from build123d import *

# Parameters (mm, degrees)
BOSS_EXTRU_1_DEPTH           = 35
ESQUISSE2_W                  = 30
ESQUISSE2_H                  = 5.1
ENL_V_MAT_EXTRU_1_DEPTH      = 10
ENL_V_MAT_EXTRU_2_DEPTH      = 38.178656511
ENL_V_MAT_EXTRU_2_DEPTH_BACK = 38.178656511
ESQUISSE3_R                  = 2.05
CONG_1_R                     = 1.5


with BuildPart() as part:
    # Esquisse1 → Boss.-Extru.1 (new body)
    with BuildSketch(Plane(origin=(0, 0, 0), x_dir=(0, 0, -1), z_dir=(1, 0, 0))):
        with BuildLine():
            Line((6, 7.5), (-6, 7.5))
            ThreePointArc((-6, 7.5), (-7.060660172, 7.060660172), (-7.5, 6))
            Line((-7.5, 6), (-7.5, -6))
            ThreePointArc((-7.5, -6), (-7.060660172, -7.060660172), (-6, -7.5))
            Line((-6, -7.5), (6, -7.5))
            ThreePointArc((6, -7.5), (7.060660172, -7.060660172), (7.5, -6))
            Line((7.5, -6), (7.5, 6))
            ThreePointArc((7.5, 6), (7.060660172, 7.060660172), (6, 7.5))
        make_face()
    extrude(amount=BOSS_EXTRU_1_DEPTH)

    # Esquisse2 → Enlèv. mat.-Extru.1 (cut)
    with BuildSketch(Plane.XY.offset(7.5)):
        with Locations((17.5, 0)):
            Rectangle(ESQUISSE2_W, ESQUISSE2_H)
    extrude(amount=-ENL_V_MAT_EXTRU_1_DEPTH, mode=Mode.SUBTRACT)

    # Esquisse3 → Enlèv. mat.-Extru.2 (cut, two sides: drawn at the far end of the back side and taken through both)
    with BuildSketch(Plane(origin=(0, -2.55, 0), x_dir=(1, 0, 0), z_dir=(0, 1, 0)).offset(-ENL_V_MAT_EXTRU_2_DEPTH_BACK)):
        with Locations(Location((9.5, -2.5, 0), (0, 0, 180))):
            Circle(ESQUISSE3_R)
        with Locations((25.5, -2.5)):
            Circle(ESQUISSE3_R)
    extrude(amount=ENL_V_MAT_EXTRU_2_DEPTH + ENL_V_MAT_EXTRU_2_DEPTH_BACK, mode=Mode.SUBTRACT)

    # Congé1
    cong_1_edges = [part.edges().sort_by_distance(p)[0] for p in [
        (0, 0, 7.5),
        (0, 7.060660172, 7.060660172),
        (0, 7.5, 0),
        (0, 7.060660172, -7.060660172),
        (35, 7.060660172, 7.060660172),
        (35, 0, 7.5),
        (35, -7.060660172, 7.060660172),
        (35, -7.5, 0),
        (35, -7.060660172, -7.060660172),
        (35, 0, -7.5),
        (35, 7.060660172, -7.060660172),
        (0, 0, -7.5),
        (35, 7.5, 0),
        (0, -7.060660172, -7.060660172),
        (0, -7.5, 0),
        (0, -7.060660172, 7.060660172),
    ]]
    fillet(cong_1_edges, radius=CONG_1_R)


solid = part.part
Design review of the part built by this model. Coordinates are the model's own, in mm. A direction names the side the tool comes from. Give positions to 0.01 mm unless a question says otherwise; leave off trailing zeros. Write each loop counter-clockwise with the first axis right and the second up, starting at its lowest first coordinate (ties: lowest second). Pieces come first, ordered by that corner, then holes. Notation, with made-up numbers: M -12,86 L 12,86 A25 ccw 12,104 Z; hole C 11,-1.5 d10. An arc over 180 degrees is marked long. Answer as a JSON object with one key per item and string values. Group by question number.
1) We need section D-D (z = 1.5). Give the boundary of the cut face in (x, y), and give its area (3 significant figures).
2) We need section A-A (z = -0.75). Give the boundary of the cut face in (x, y), and give its area (3 significant figures).
3) For line 1 along Z through (x, y) = (25.5, 5.35); line 2 along Y through (x, z) = (17, 4); line 3 along X through (y, z) = (6.25, 2.75), list the stretches that pass through material, from the lowest coordinate up.
4) Mouldability with a two-part tool opening along Y and no side actions: class faces 3 (the face through (17, 2.55, 3)), 4 (the face through (0.43, -0.08, 7.05)), 5 (the face through (17.28, 7.07, 7.05)) as released by +Y, released by -Y, zero draft, split by the parting line, or undercut.
5) We need section C-C (x = 9.5). Give the boundary of the cut face in (y, z).
6) Tool access review of faces 1 (the face through (17, -2.55, 3)), 2 (the face through (17, 0, -7.5)): name each direction out of +Z, -Z, +X, -X, +Y, -Y from which nothing blocks a thin tool from reaching the whole face with its end or side.
7) Clearance check with a flat-ended pin moving along its axis: pin 1 Ø3 at (x, y) = (21.5, 0.5) entering from +Z. State where the tip first meets the part, or that it passes through.
8) We need section B-B (y = 3). Give the boundary of the cut face in (x, z), and give its area (3 significant figures).
Answer key:
{
 "1": {"outline": "M 0,-6 A1.5 ccw 1.5,-7.5 L 7.71,-7.5 L 7.71,-2.55 L 2.5,-2.55 L 2.5,2.55 L 7.71,2.55 L 7.71,7.5 L 1.5,7.5 A1.5 ccw 0,6 Z; M 11.29,-7.5 L 23.71,-7.5 L 23.71,-2.55 L 11.29,-2.55 Z; M 11.29,2.55 L 23.71,2.55 L 23.71,7.5 L 11.29,7.5 Z; M 27.29,-7.5 L 33.5,-7.5 A1.5 ccw 35,-6 L 35,6 A1.5 ccw 33.5,7.5 L 27.29,7.5 L 27.29,2.55 L 32.5,2.55 L 32.5,-2.55 L 27.29,-2.55 Z", "area": "299 mm²"},
 "2": {"outline": "M 0,-6 A1.5 ccw 1.5,-7.5 L 33.5,-7.5 A1.5 ccw 35,-6 L 35,6 A1.5 ccw 33.5,7.5 L 1.5,7.5 A1.5 ccw 0,6 Z; hole M 2.5,-2.55 L 32.5,-2.55 L 32.5,2.55 L 2.5,2.55 Z", "area": "370 mm²"},
 "3": {"line 1": "z = -7.5 to 0.45, 4.55 to 7.5", "line 2": "y = -7.5 to -2.55, 2.55 to 7.5", "line 3": "x = 0.02 to 7.47, 11.53 to 23.47, 27.53 to 34.98"},
 "4": {"face 3": "undercut", "face 4": "zero draft", "face 5": "released by +Y"},
 "5": {"outline": "M -7.5,-6 A1.5 ccw -6,-7.5 L 6,-7.5 A1.5 ccw 7.5,-6 L 7.5,0.45 L 2.55,0.45 L 2.55,-2.5 L -2.55,-2.5 L -2.55,0.45 L -7.5,0.45 Z; M -7.5,4.55 L -2.55,4.55 L -2.55,7.5 L -6,7.5 A1.5 ccw -7.5,6 Z; M 2.55,4.55 L 7.5,4.55 L 7.5,6 A1.5 ccw 6,7.5 L 2.55,7.5 Z"},
 "6": {"face 1": "+Z", "face 2": "-Z, +X, -X, +Y, -Y"},
 "7": {"pin 1": "stops at z = -2.5"},
 "8": {"outline": "M 0,-6 A1.5 ccw 1.5,-7.5 L 33.5,-7.5 A1.5 ccw 35,-6 L 35,6 A1.5 ccw 33.5,7.5 L 1.5,7.5 A1.5 ccw 0,6 Z; hole C 9.5,2.5 d4.1; hole C 25.5,2.5 d4.1", "area": "497 mm²"}
}
